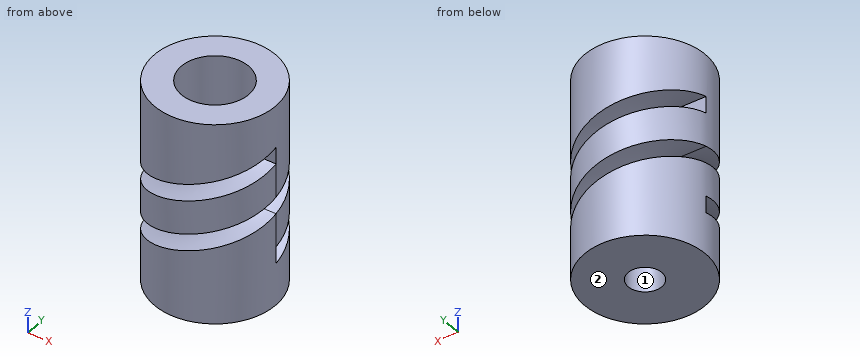
Autodesk Inventor part; units mm, degrees
ref_plane "YZ Plane" through (0, 0, 0) normal (1, 0, 0) x (0, 1, 0)
ref_plane "XZ Plane" through (0, 0, 0) normal (0, 1, 0) x (-1, 0, 0)
ref_plane "XY Plane" through (0, 0, 0) normal (0, 0, 1) x (1, 0, 0)
sketch "Sketch1" plane through (0, 0, 0) normal (0, 0, 1) x (1, 0, 0)
  circle A0 centre (0, 0) radius 9
  circle A1 centre (0, 0) radius 2.5
  dimension "d0" = 18
  dimension "d3" = 5
extrude "Extrusion1" add sketch "Sketch1" along normal blind 30
sketch "Sketch2" plane through (0, 0, 30) normal (0, 0, 1) x (1, 0, 0)
  circle A0 centre (0, 0) radius 2.5
  circle A1 centre (0, 0) radius 9
  circle A2 centre (0, 0) radius 5
  dimension "d4" = 10
extrude "Extrusion2" cut sketch "Sketch2" against normal blind 20 contours A2
sketch "Sketch3" plane through (0, 0, 0) normal (0, 1, 0) x (-1, 0, 0)
  line L0 (9, 30) -> (9, 0)
  line L1 (9, 0) -> (2.5, 0)
  line L2 (2.5, 0) -> (2.5, 10)
  line L3 (2.5, 10) -> (5, 10)
  line L4 (5, 10) -> (5, 30)
  line L5 (5, 30) -> (9, 30)
  line L6 (-9, 0) -> (-9, 30)
  line L7 (-9, 30) -> (-5, 30)
  line L8 (-5, 30) -> (-5, 10)
  line L9 (-5, 10) -> (-2.5, 10)
  line L10 (-2.5, 10) -> (-2.5, 0)
  line L11 (-2.5, 0) -> (-9, 0)
  line L12 (0, 0) -> (9, 0)
  line L13 (9, 0) -> (9, 30)
  line L14 (9, 30) -> (0, 30)
  line L15 (0, 30) -> (0, 0)
  line L16 (-9, 6.25) -> (-5, 6.25)
  line L17 (-5, 6.25) -> (-5, 8.75)
  line L18 (-5, 8.75) -> (-9, 8.75)
  line L19 (-9, 8.75) -> (-9, 6.25)
  line L20 (-9, 15) -> (0, 15) construction
  line L21 (-9, 7.5) -> (-5, 7.5) construction
  dimension "d20" = 2.5
  dimension "d22" = 7.5
extrude "Extrusion3" [suppressed]
coil "Coil1" sketch "Sketch3" operation cut axis through (0, 0, -10) along (0, 0, 1) pitch 15 turns 1 hand right contours L6 L18 L17 L16
pattern_circular "Circular Pattern1" count 2 over 360 about axis through (0, 0, -10) along (0, 0, 1) of "Coil1"
properties part number "z-coupler"
Design review of the part built by this model. Coordinates are the model's own, in mm. Face numbers are marked on the shaded views. Round coordinates to 2 decimals unless told otherwise and drop trailing zeros. Loops run counter-clockwise (first coordinate to the right, second up) from the corner with the lowest first, then second, coordinate; pieces in that order, holes last. Notation, with made-up numbers: (61, 3) - (116, 3) arc R23 cw to (116, 19) - close; hole circle Ø6 at (16, 2). An arc over 180 degrees is marked (long way). One line per item, written item: value. Start each with the question number.
1) To check wall thickness, follow L1, parallel to Z at x = -4.75, y = 3.5; L2, parallel to Y at x = 0, z = 14. State the ranges of each line that lie inside material, in increasing order. Write a range as from..to.
2) Draft analysis for pull direction X (two halves, no side actions). For the marked faces 1 and 2, state which applies: +X half, -X half, draft (parallel to the pull), parting line (faces both ways), or undercut.
3) Consider section A-A on z = 4.5. Give the boundary of the cut face in (x, y).
4) Insertion check: pin 1 Ø3 at (x, z) = (5.5, 16) entering from -Y; pin 2 Ø0.8 at (x, z) = (6.5, 22) entering from -Y; pin 3 Ø4 at (x, z) = (5, 11.5) entering from +Y. Each pin has a flat end and moves straight along its axis. Give the tip position at first contact, or say it passes through.
5) Consider section B-B on x = 0.75. Give the number of separate pieces and of enclosed holes in the cut face, then the cut area to 3 significant figures.
Reported:
1. L1: z = 0..12.23, 14.73..19.73, 22.23..30
1. L2: y = -9..-5, 5..9
2. face 1: undercut
2. face 2: draft
3. outline: circle Ø18 at (0, 0); hole circle Ø5 at (0, 0)
4. pin 1: stops at y = -8.06
4. pin 2: stops at y = -6.62
4. pin 3: stops at y = 8.48
5. separate pieces: 6
5. enclosed holes: 0
5. area: 252 mm^2
